For this review, take the finished solid that the model builds, in its own axes (mm). Round coordinates to 2 decimals unless told otherwise and drop trailing zeros. Order: outer loops, then holes, each group sorted by start corner. A loop starts at its lowest first (then second) coordinate and runs counter-clockwise, first axis right, second up. Notation, with made-up numbers: (-2.75, 8.5) - (3.25, 8.5) arc R19 ccw to (3.25, 40.5) - close; hole circle Ø1 at (37.25, 62). An arc over 180 degrees is marked (long way). One line per item, written item: value.
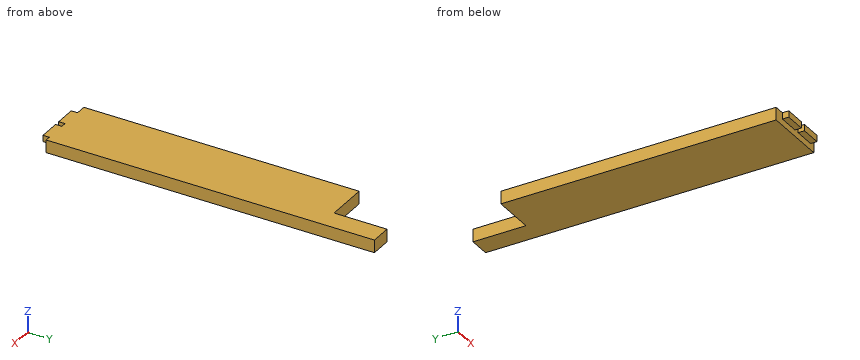
Autodesk Inventor part; units mm, degrees
ref_plane "YZ Plane" through (0, 0, 0) normal (1, 0, 0) x (0, 1, 0)
ref_plane "XZ Plane" through (0, 0, 0) normal (0, 1, 0) x (-1, 0, 0)
ref_plane "XY Plane" through (0, 0, 0) normal (0, 0, 1) x (1, 0, 0)
sketch "Sketch1" plane through (0, 0, 0) normal (0, 0, 1) x (1, 0, 0)
  line L0 (0, 266) -> (0, 6)
  line L1 (60, 6) -> (60, 316)
  line L2 (0, 6) -> (10, 6)
  line L3 (10, 6) -> (10, 0)
  line L4 (10, 0) -> (30, 0)
  line L5 (30, 0) -> (30, 6)
  line L6 (30, 6) -> (35, 6)
  line L7 (35, 6) -> (35, 0)
  line L8 (35, 0) -> (55, 0)
  line L9 (55, 0) -> (55, 6)
  line L10 (55, 6) -> (60, 6)
  line L11 (60, 316) -> (40, 316)
  line L12 (40, 316) -> (40, 266)
  line L13 (40, 266) -> (0, 266)
  point P0 (0, 0)
  dimension "d25" = 10
  dimension "d26" = 20
  dimension "d27" = 5
  dimension "d29" = 20
  dimension "d31" = 310
  dimension "d32" = 20
  dimension "d33" = 50
  dimension "d34" = 6
extrude "Extrusion1" add sketch "Sketch1" against normal blind 6
sketch "Sketch3" plane through (0, 0, -6) normal (0, 0, -1) x (-1, 0, 0)
  line L0 (-60, 316) -> (-60, 6)
  line L1 (-60, 316) -> (-60, 6)
  line L2 (-60, 6) -> (0, 6)
  line L3 (-40, 316) -> (-60, 316)
  line L4 (0, 6) -> (0, 266)
  line L5 (0, 6) -> (0, 266)
  line L6 (0, 266) -> (-40, 266)
  line L7 (-40, 266) -> (-40, 316)
  line L8 (-40, 266) -> (-40, 316)
  point P0 (0, 0)
extrude "Extrusion3" add sketch "Sketch3" along normal blind 6
properties part number "Archimedes Screw Border3"
Item 1: Wall thickness on line 1 (Y direction, x = 52, z = -7.25); line 2 (Y direction, x = 15, z = -2.5); line 3 (X direction, y = 300, z = -5.75): over which ranges is each line inside the solid? List them lowest first.
Returned:
line 1: 6 to 316
line 2: 0 to 266
line 3: 40 to 60
Item 2: Take a section at B-B (x = 16). Write out the cut boundary in (y, z), plus the area to 3 significant figures.
Returned:
outline: (0, -6) - (6, -6) - (6, -12) - (266, -12) - (266, 0) - (0, 0) - close
area: 3,160 mm^2
Item 3: Take a section at A-A (z = -2.5). Write out the cut boundary in (x, y), plus the area to 3 significant figures.
Returned:
outline: (0, 6) - (10, 6) - (10, 0) - (30, 0) - (30, 6) - (35, 6) - (35, 0) - (55, 0) - (55, 6) - (60, 6) - (60, 316) - (40, 316) - (40, 266) - (0, 266) - close
area: 16,800 mm^2
Item 4: Take a section at C-C (y = 272). Write out the cut boundary in (x, z).
Returned:
outline: (40, -12) - (60, -12) - (60, 0) - (40, 0) - close
Item 5: For P1, Ø1, axis at x = 33, z = -5.5, coming from the +Y side; P2, Ø3, axis at x = 41.5, y = 2, coming from the -Z side; P3, Ø3, axis at y = 2.5, z = -3, coming from the +X side, all flat-tipped, find the tip position at first contact; note any pin that passes through.
Returned:
P1: y = 266
P2: z = -6
P3: x = 55
